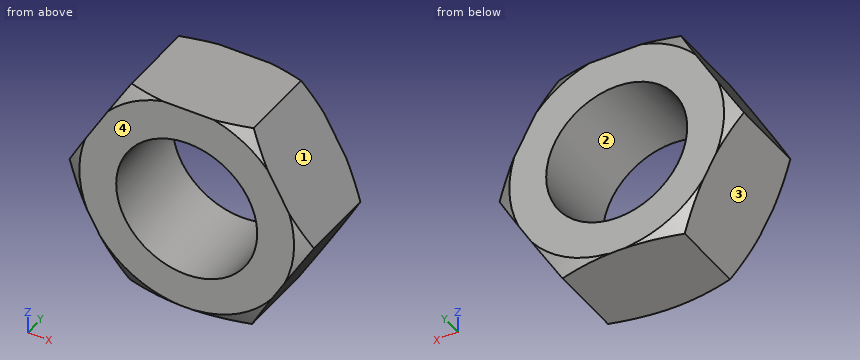
```python
from build123d import *

# Parameters (mm, degrees)
F1_DEPTH = 10.7188
F2_R     = 7.9375
F3_DEPTH = 10.7198


with BuildPart() as f1:
    # F0 (on Front) → F1 (new body)
    with BuildSketch(Plane.XZ):
        Polygon((-13.754363, 0.175734), (-7.029372, -11.823761), (6.724991, -11.999495), (13.754363, -0.175734), (7.029372, 11.823761), (-6.724991, 11.999495), align=None)
    extrude(amount=F1_DEPTH)

    # F2 (on face) → F3 (cut, through all)
    with BuildSketch(Plane.XZ.offset(10.7188)):
        Circle(F2_R)
    extrude(amount=-F3_DEPTH, mode=Mode.SUBTRACT)

    # F4 (on Right) → F5 (revolve, cut)
    with BuildSketch(Plane.YZ):
        Polygon((-6.554505, -19.124399), (-10.7188, -11.911628), (-10.7188, -19.124399), align=None)
        Polygon((0, -11.911628), (-4.164295, -19.124399), (0, -19.124399), align=None)
    revolve(axis=Axis((0, -5.3594, 0.175734), (0, -1, 0)), mode=Mode.SUBTRACT)


solid = f1.part
```
Can you work these out from the model? Positions are in its coordinate system, mm. Face numbers are marked on the shaded views. Give positions to 0.01 mm unless a question says otherwise; leave off trailing zeros. Loops run counter-clockwise (first coordinate to the right, second up) from the corner with the lowest first, then second, coordinate; pieces in that order, holes last. Notation, with made-up numbers: M 62,-10 L 92,-10 A18 ccw 92,10 Z; hole C 74.25,50 d11. An arc over 180 degrees is marked long. Use CSV: the item, a comma, the result in double quotes. Start each with the question number.
1. Imagine slicing it at B-B, the plane z = -6.25. Write out the boundary of the cut face in (x, y).
2. If I drill on L1, parallel to X at y = -8.5, z = 4.75; L2, parallel to Z at x = 0, y = -4.75; L3, parallel to X at y = -2.75, z = -7, over which ranges is the centre line in solid material (lowest first)?
3. For P1, Ø5, axis at y = -9, z = 7.5, coming from the -X side; P2, Ø1, axis at y = -7, z = -2.5, coming from the -X side (3 decimals); P3, Ø8, axis at x = -0.5, z = 7, coming from the -Y side, each with a flat end and sliding along its axis, tell me the tip position at first contact or that it passes through.
4. Imagine slicing it at A-A, the plane y = -4. Write out the boundary of the cut face in (x, z) (1 decimal), plus the area to 3 significant figures.
5. If we mould it in two halves opening along X, with no side actions, what happens to the marked faces 1, 2, 3 and 4? For each: released by +X, released by -X, zero draft, split by the parting line, or undercut.
Response values:
1,outline,"M -10.15,-10.72 L -4.89,-10.72 L -4.89,0 L -10.15,0 Z; M 4.89,-10.72 L 10.14,-10.72 L 10.14,0 L 4.89,0 Z"
2,L1,"-11.03 to -6.36, 6.36 to 10.99"
2,L2,"-11.91 to -7.94, 7.94 to 11.91"
2,L3,"-9.73 to -3.74, 3.74 to 9.7"
3,P1,"x = -10.89"
3,P2,"x = -12.535"
3,P3,"y = -10.72"
4,outline,"M -13.8,0.2 L -7,-11.8 L 6.7,-12 L 13.8,-0.2 L 7,11.8 L -6.7,12 Z; hole C 0,0 d15.9"
4,area,"294 mm^2"
5,face 1,"released by +X"
5,face 2,"undercut"
5,face 3,"released by -X"
5,face 4,"zero draft"
